from build123d import *

# Parameters (mm, degrees)
SKETCH_1_R               = 19
EXTRUDE_1_DEPTH          = 20
EXTRUDE_2_DEPTH          = 3
SKETCH_6_R               = 17
CUT_EXTRUDE_1_DEPTH      = 18
SKETCH_7_R               = 17
SKETCH_7_R_2             = 15
EXTRUDE_3_DEPTH          = 9.5
CUT_EXTRUDE_2_REACH      = 44.629
SKETCH_8_R               = 13
EXTRUDE_START            = -2
EXTRUDE_4_DEPTH          = 2
HOLE_WIZARD_M3_1_D       = 2.5
HOLE_WIZARD_M3_1_DEPTH   = 3
HOLE_WIZARD_M2_1_D       = 1.6
CUT_EXTRUDE_3_DEPTH      = 44.800684926
CUT_EXTRUDE_3_DEPTH_BACK = 44.800684926
SKETCH_17_W              = 74
SKETCH_17_H              = 33
SKETCH_18_R              = 15
SKETCH_18_R_2            = 6
EXTRUDE_5_DEPTH          = 2


with BuildPart() as part:
    # 草图1 → 凸台-拉伸1 (new body)
    with BuildSketch(Plane.XY):
        Circle(SKETCH_1_R)
    extrude(amount=EXTRUDE_1_DEPTH)

    # 草图3 → 凸台-拉伸2 (add)
    with BuildSketch(Plane.XY.offset(20)):
        with BuildLine():
            Line((-22.5, 10), (22.5, 10))
            ThreePointArc((22.5, 10), (32.5, 0), (22.5, -10))
            Line((22.5, -10), (-22.5, -10))
            ThreePointArc((-22.5, -10), (-32.5, 0), (-22.5, 10))
        make_face()
    extrude(amount=-EXTRUDE_2_DEPTH)

    # 草图6 → 切除-拉伸1 (cut)
    with BuildSketch(Plane.XY.offset(20)):
        Circle(SKETCH_6_R)
    extrude(amount=-CUT_EXTRUDE_1_DEPTH, mode=Mode.SUBTRACT)

    # 草图7 → 凸台-拉伸3 (add)
    with BuildSketch(Plane(origin=(0, 0, 0), x_dir=(-1, 0, 0), z_dir=(0, 0, -1))):
        with Locations(Location((0, 0, 0), (0, 0, 180))):
            Circle(SKETCH_7_R)
        Circle(SKETCH_7_R_2, mode=Mode.SUBTRACT)
    extrude(amount=EXTRUDE_3_DEPTH)

    # 草图8 → 切除-拉伸2 (cut, up to next)
    with BuildSketch(Plane(origin=(0, 0, 0), x_dir=(-1, 0, 0), z_dir=(0, 0, -1)), mode=Mode.PRIVATE) as cut_extrude_2_sk1:
        Circle(SKETCH_8_R)
    cut_extrude_2_tool1 = extrude(cut_extrude_2_sk1.sketch, amount=-CUT_EXTRUDE_2_REACH, mode=Mode.PRIVATE) & part.part
    add(cut_extrude_2_tool1.solids().sort_by_distance((0, 0, 0))[0], mode=Mode.SUBTRACT)

    # 草图10 → 凸台-拉伸4 (add)
    with BuildSketch(Plane(origin=(0, 0, -9.5), x_dir=(-1, 0, 0), z_dir=(0, 0, -1)).offset(EXTRUDE_START)):
        with BuildLine():
            Line((-16.815171721, 2.5), (-23.815171721, 2.5))
            ThreePointArc((-23.815171721, 2.5), (-26.315171721, 0), (-23.815171721, -2.5))
            Line((-23.815171721, -2.5), (-16.815171721, -2.5))
            ThreePointArc((-16.815171721, -2.5), (-17, 0), (-16.815171721, 2.5))
        make_face()
        with BuildLine():
            Line((16.815171721, 2.5), (23.815171721, 2.5))
            ThreePointArc((23.815171721, 2.5), (26.315171721, 0), (23.815171721, -2.5))
            Line((23.815171721, -2.5), (16.815171721, -2.5))
            ThreePointArc((16.815171721, -2.5), (17, 0), (16.815171721, 2.5))
        make_face()
    extrude(amount=EXTRUDE_4_DEPTH)

    # M3 螺纹孔的螺纹孔钻头1
    with Locations(Plane(origin=(0, 0, 17), x_dir=(-1, 0, 0), z_dir=(0, 0, -1))):
        with Locations((-23.815171721, 0)):
            hole_wizard_m3_1 = Hole(HOLE_WIZARD_M3_1_D / 2, depth=HOLE_WIZARD_M3_1_DEPTH)

    # M2 螺纹孔的螺纹孔钻头1 (through all)
    with Locations(Plane(origin=(0, 0, -9.5), x_dir=(-1, 0, 0), z_dir=(0, 0, -1))):
        with Locations((-23.815171721, 0)):
            hole_wizard_m2_1 = Hole(HOLE_WIZARD_M2_1_D / 2)

    # 镜向1: M3 螺纹孔的螺纹孔钻头1, M2 螺纹孔的螺纹孔钻头1 across plane
    add(hole_wizard_m3_1.mirror(Plane(origin=(0, 0, 0), x_dir=(0, 0, 1), z_dir=(1, 0, 0))), mode=Mode.SUBTRACT)
    add(hole_wizard_m2_1.mirror(Plane(origin=(0, 0, 0), x_dir=(0, 0, 1), z_dir=(1, 0, 0))), mode=Mode.SUBTRACT)

    # 草图17 → 切除-拉伸3 (cut, two sides: drawn at the far end of the back side and taken through both)
    with BuildSketch(Plane.XZ.offset(2.5).offset(-CUT_EXTRUDE_3_DEPTH_BACK)):
        with Locations((0, 9)):
            Rectangle(SKETCH_17_W, SKETCH_17_H)
    extrude(amount=CUT_EXTRUDE_3_DEPTH + CUT_EXTRUDE_3_DEPTH_BACK, mode=Mode.SUBTRACT)

    # 草图18 → 凸台-拉伸5 (add)
    with BuildSketch(Plane(origin=(0, 0, -9.5), x_dir=(-1, 0, 0), z_dir=(0, 0, -1)).offset(EXTRUDE_START)):
        Circle(SKETCH_18_R)
        Circle(SKETCH_18_R_2, mode=Mode.SUBTRACT)
    extrude(amount=EXTRUDE_5_DEPTH)


solid = part.part
Model file for the job. Use its own axes, mm. A direction names the side the tool comes from. Coordinates: 2 decimals unless noted, no trailing zeros. Order: outer loops, then holes, each group sorted by start corner. A loop starts at its lowest first (then second) coordinate and runs counter-clockwise, first axis right, second up. Notation, with made-up numbers: (-15, 35) -> (-3, 35) arc R29 ccw to (-3, 63) -> close; hole circle Ø7 at (54, -30.5). An arc over 180 degrees is marked (long way). Return JSON: item names as keys, results as strings. Group by question number.
Item 1: Wall check: line 1 along Y through (x, z) = (0, -8.45); line 2 along Y through (x, z) = (21, -8.1); line 3 along Y through (x, z) = (-3.5, -8). Give the ranges that are in metal, low to high. Write a range as [from, to].
Item 2: Saw through at C-C on x = 0. Write the cut outline in (y, z), then the cut area to 3 significant figures.
Item 3: Flat gauge pins, fed straight in: P1, Ø2, axis at x = -23.82, y = 0, coming from the -Z side; P2, Ø0.6, axis at x = -20.5, z = -8.5, coming from the +Y side; P3, Ø0.6, axis at x = -19, z = -8.5, coming from the -Y side. Where does each tip first touch, or does it go through?
Item 4: Pull direction Y, two halves, no side cores. Call faces 4 (the flat face through (6.2, 0.2, -9.5)), 5 (the cylindrical face through (6, 0, -8)), 6 (the cylindrical face through (-26.315, 0.055, -8.486)), 7 (the flat face through (-20, 2.5, -8)): pulls with the +Y half, pulls with the -Y half, needs draft (parallel to the pull), parting line crosses it, or undercut.
Item 5: Saw through at B-B on z = -8. Write the cut outline in (x, y).
Item 6: Tool access for faces 1 (the flat face through (20, 2.5, -8)), 2 (the flat face through (-20, -2.5, -8)), 3 (the flat face through (20, -2.5, -8)): list every direction of +Z, -Z, +X, -X, +Y, -Y with a clear straight run to the whole face (end or side of a thin tool).
Item 7: Saw through at D-D on y = -8. Write the cut outline in (x, z), then the cut area to 3 significant figures.
Item 8: Saw through at A-A on y = 0. Write the cut outline in (x, z).
Values found:
{
 "1": {"line 1": "y = [-17, -6], [6, 17]", "line 2": "y = [-2.5, 2.5]", "line 3": "y = [-16.64, -4.87], [4.87, 16.64]"},
 "2": {"outline": "(-17, -9.5) -> (-6, -9.5) -> (-6, -7.5) -> (-17, -7.5) -> close; (6, -9.5) -> (17, -9.5) -> (17, -7.5) -> (6, -7.5) -> close", "area": "44.0 mm2"},
 "3": {"P1": "stops at z = -9.5", "P2": "stops at y = 2.5", "P3": "stops at y = -2.5"},
 "4": {"face 4": "needs draft", "face 5": "undercut", "face 6": "parting line crosses it", "face 7": "pulls with the +Y half"},
 "5": {"outline": "(-23.82, -2.5) -> (-16.82, -2.5) arc R17 ccw to (16.82, -2.5) -> (23.82, -2.5) arc R2.5 ccw to (23.82, 2.5) -> (16.82, 2.5) arc R17 ccw to (-16.82, 2.5) -> (-23.82, 2.5) arc R2.5 ccw to start; hole circle Ø1.6 at (-23.82, 0); hole circle Ø12 at (0, 0); hole circle Ø1.6 at (23.82, 0)"},
 "6": {"face 1": "+Z, -Z, +X, +Y", "face 2": "+Z, -Z, -X, -Y", "face 3": "+Z, -Z, +X, -Y"},
 "7": {"outline": "(-15, -9.5) -> (15, -9.5) -> (15, -7.5) -> (-15, -7.5) -> close", "area": "60.0 mm2"},
 "8": {"outline": "(-26.32, -9.5) -> (-24.62, -9.5) -> (-24.62, -7.5) -> (-26.32, -7.5) -> close; (-23.02, -9.5) -> (-6, -9.5) -> (-6, -7.5) -> (-23.02, -7.5) -> close; (6, -9.5) -> (23.02, -9.5) -> (23.02, -7.5) -> (6, -7.5) -> close; (24.62, -9.5) -> (26.32, -9.5) -> (26.32, -7.5) -> (24.62, -7.5) -> close"}
}
